```python
from build123d import *

# Parameters (mm, degrees)
BASE_FLANGE1_START             = -3.175
BASE_FLANGE1_OUTLINE_W         = 1184.91
BASE_FLANGE1_OUTLINE_H         = 203.2
BASE_FLANGE1_DEPTH             = 6.35
EDGE_FLANGE1_STRIP_W           = 48.1
EDGE_FLANGE1_STRIP_H           = 6.35
EDGE_FLANGE1_STRIP_CUT_DEPTH   = 203.2
EDGE_FLANGE1_STRIP_2_W         = 48.1
EDGE_FLANGE1_STRIP_2_H         = 6.35
EDGE_FLANGE1_STRIP_CUT_2_DEPTH = 203.2
EDGE_FLANGE1_DEPTH             = 203.2
EDGE_FLANGE1_BEND_DEPTH        = 203.2
BOSS_EXTRUDE1_START            = -6.35
BOSS_EXTRUDE1_DEPTH            = 6.35
CUT_EXTRUDE1_REACH             = 1310.867
SKETCH13_R                     = 38.1
SKETCH13_W                     = 25.908
SKETCH13_H                     = 27.94
BOSS_EXTRUDE2_DEPTH            = 6.35
MIRROR3_START                  = -165.354
MIRROR3_OUTLINE_W              = 6.35
MIRROR3_OUTLINE_H              = 27.94
MIRROR3_DEPTH                  = 25.908
MIRROR3_START_2                = 139.446
MIRROR3_2_OUTLINE_W            = 6.35
MIRROR3_2_OUTLINE_H            = 27.94
MIRROR3_2_DEPTH                = 25.908


# Read off the part's stored shape, not the designer's step: Base-Flange1, Mirror3
# Sheet-metal steps are written as plain solids
with BuildPart() as part:
    # Base-Flange1 outline → Base-Flange1 (new body)
    with BuildSketch(Plane(origin=(0, 0, 0), x_dir=(1, 0, 0), z_dir=(0, 1, 0)).offset(BASE_FLANGE1_START)):
        Rectangle(BASE_FLANGE1_OUTLINE_W, BASE_FLANGE1_OUTLINE_H)
    extrude(amount=BASE_FLANGE1_DEPTH)

    # Edge-Flange1 strip (across the edge) → Edge-Flange1 strip cut (cut)
    with BuildSketch(Plane(origin=(592.455, -3.175, -101.6), x_dir=(-1, 0, 0), z_dir=(0, 0, 1))):
        with Locations((-11.35, -3.175)):
            Rectangle(EDGE_FLANGE1_STRIP_W, EDGE_FLANGE1_STRIP_H)
    extrude(amount=EDGE_FLANGE1_STRIP_CUT_DEPTH, mode=Mode.SUBTRACT)

    # Edge-Flange1 strip 2 (across the edge) → Edge-Flange1 strip cut 2 (cut)
    with BuildSketch(Plane(origin=(-592.455, -3.175, 101.6), x_dir=(1, 0, 0), z_dir=(0, 0, -1))):
        with Locations((-11.35, -3.175)):
            Rectangle(EDGE_FLANGE1_STRIP_2_W, EDGE_FLANGE1_STRIP_2_H)
    extrude(amount=EDGE_FLANGE1_STRIP_CUT_2_DEPTH, mode=Mode.SUBTRACT)

    # Edge-Flange1 section (across the edge) → Edge-Flange1 (add)
    with BuildSketch(Plane(origin=(592.455, -3.175, -101.6), x_dir=(-1, 0, 0), z_dir=(0, 0, 1))):
        with BuildLine():
            Line((0, 6.35), (0, 514.35))
            Line((0, 514.35), (6.35, 514.35))
            Line((6.35, 514.35), (6.35, 6.35))
            ThreePointArc((6.35, 6.35), (8.209871939, 1.859871939), (12.7, 0))
            Line((12.7, 0), (12.7, -6.35))
            ThreePointArc((12.7, -6.35), (3.719743879, -2.630256121), (0, 6.35))
        make_face()
    extrude(amount=EDGE_FLANGE1_DEPTH)

    # Edge-Flange1 section 2 (across the edge) → Edge-Flange1 bend (add)
    with BuildSketch(Plane(origin=(-592.455, -3.175, 101.6), x_dir=(1, 0, 0), z_dir=(0, 0, -1))):
        with BuildLine():
            Line((0, 6.35), (0, 514.35))
            Line((0, 514.35), (6.35, 514.35))
            Line((6.35, 514.35), (6.35, 6.35))
            ThreePointArc((6.35, 6.35), (8.209871939, 1.859871939), (12.7, 0))
            Line((12.7, 0), (12.7, -6.35))
            ThreePointArc((12.7, -6.35), (3.719743879, -2.630256121), (0, 6.35))
        make_face()
    extrude(amount=EDGE_FLANGE1_BEND_DEPTH)

    # Sketch12 → Boss-Extrude1 (add)
    with BuildSketch(Plane(origin=(592.455, 0, 0), x_dir=(0, 0, -1), z_dir=(1, 0, 0)).offset(BOSS_EXTRUDE1_START)):
        Polygon((-101.6, -238.125), (-203.2, -339.725), (-203.2, -517.525), (-101.6, -517.525), align=None)
        Polygon((203.2, -339.725), (101.6, -238.125), (101.6, -517.525), (203.2, -517.525), align=None)
    extrude(amount=BOSS_EXTRUDE1_DEPTH)

    # Sketch13 → Cut-Extrude1 (cut, up to next)
    with BuildSketch(Plane(origin=(592.455, 0, 0), x_dir=(0, 0, -1), z_dir=(1, 0, 0)), mode=Mode.PRIVATE) as cut_extrude1_sk1:
        with Locations(Location((0, -73.025, 0), (0, 0, 90))):
            Circle(SKETCH13_R)
    cut_extrude1_tool1 = extrude(cut_extrude1_sk1.sketch, amount=-CUT_EXTRUDE1_REACH, mode=Mode.PRIVATE) & part.part
    # Sketch13 → Cut-Extrude1 (cut, up to next)
    with BuildSketch(Plane(origin=(592.455, 0, 0), x_dir=(0, 0, -1), z_dir=(1, 0, 0)), mode=Mode.PRIVATE) as cut_extrude1_sk2:
        with Locations((152.4, -475.107)):
            Rectangle(SKETCH13_W, SKETCH13_H)
    cut_extrude1_tool2 = extrude(cut_extrude1_sk2.sketch, amount=-CUT_EXTRUDE1_REACH, mode=Mode.PRIVATE) & part.part
    # Sketch13 → Cut-Extrude1 (cut, up to next)
    with BuildSketch(Plane(origin=(592.455, 0, 0), x_dir=(0, 0, -1), z_dir=(1, 0, 0)), mode=Mode.PRIVATE) as cut_extrude1_sk3:
        with Locations((-152.4, -475.107)):
            Rectangle(SKETCH13_W, SKETCH13_H)
    cut_extrude1_tool3 = extrude(cut_extrude1_sk3.sketch, amount=-CUT_EXTRUDE1_REACH, mode=Mode.PRIVATE) & part.part
    cut_extrude1_1 = cut_extrude1_tool1.solids().sort_by_distance((592.455, -73.025, 0))[0]
    add(cut_extrude1_1, mode=Mode.SUBTRACT)
    cut_extrude1_2 = cut_extrude1_tool2.solids().sort_by_distance((592.455, -475.107, -152.4))[0]
    add(cut_extrude1_2, mode=Mode.SUBTRACT)
    cut_extrude1_3 = cut_extrude1_tool3.solids().sort_by_distance((592.455, -475.107, 152.4))[0]
    add(cut_extrude1_3, mode=Mode.SUBTRACT)
    cut_extrude1 = cut_extrude1_1 + cut_extrude1_2 + cut_extrude1_3  # Cut-Extrude1 as one shape, for the pattern or mirror that repeats it

    # Mirror1: Cut-Extrude1 across plane
    add(cut_extrude1.mirror(Plane(origin=(0, 0, 0), x_dir=(0, 0, 1), z_dir=(1, 0, 0))), mode=Mode.SUBTRACT)

    # Sketch14 → Boss-Extrude2 (add)
    with BuildSketch(Plane.ZY.offset(592.455)):
        Polygon((203.2, -517.525), (203.2, -339.725), (101.6, -238.125), (-101.6, -238.125), (-203.2, -339.725), (-203.2, -517.525), align=None)
    extrude(amount=-BOSS_EXTRUDE2_DEPTH)

    # Mirror3 outline → Mirror3 (cut)
    with BuildSketch(Plane.XY.offset(MIRROR3_START)):
        with Locations((-589.28, -475.107)):
            Rectangle(MIRROR3_OUTLINE_W, MIRROR3_OUTLINE_H)
    extrude(amount=MIRROR3_DEPTH, mode=Mode.SUBTRACT)

    # Mirror3 2 outline → Mirror3 2 (cut)
    with BuildSketch(Plane.XY.offset(MIRROR3_START_2)):
        with Locations((-589.28, -475.107)):
            Rectangle(MIRROR3_2_OUTLINE_W, MIRROR3_2_OUTLINE_H)
    extrude(amount=MIRROR3_2_DEPTH, mode=Mode.SUBTRACT)


solid = part.part
```
Here's how the part is built. I have some questions about the finished solid (model axes, mm). A direction names the side the tool comes from. Round coordinates to 2 decimals unless told otherwise and drop trailing zeros. Order: outer loops, then holes, each group sorted by start corner. A loop starts at its lowest first (then second) coordinate and runs counter-clockwise, first axis right, second up. Notation, with made-up numbers: (-12.75, 80.5) -> (9.25, 80.5) arc R14 ccw to (9.25, 97.5) -> close; hole circle Ø9 at (43, 71.5). An arc over 180 degrees is marked (long way). Use a Markdown table: item, result. Add a question column.
(1) For pin 1 Ø3 at (x, z) = (588.5, 146) entering from +Y (3 decimals); pin 2 Ø3 at (x, z) = (207, -97) entering from -Y (3 decimals); pin 3 Ø1.9 at (x, z) = (588.5, -151) entering from +Y (3 decimals), each with a flat end and sliding along its axis, tell me the tip position at first contact or that it passes through.
(2) Suppose I cut it at D-D, the plane z = 59. Please give me the cut outline in (x, y) (3 decimals).
(3) Suppose I cut it at A-A, the plane y = -475. Please give me the cut outline in (x, z) (3 decimals), and give its area (3 significant figures).
(4) If we mould it in two halves opening along Z, with no side actions, what happens to faces 3 (the face through (589.324, -111.088, 1.675)), 4 (the face through (-8, -3.175, -1)), 5 (the face through (-589.324, -288.214, -151.689))? For each: released by +Z, released by -Z, zero draft, split by the parting line, or undercut.
(5) For faces 1 (the face through (592.455, -316, 3)), 2 (the face through (-586.105, -316, -3)), which set-ups out of +Z, -Z, +X, -X, +Y, -Y let a thin tool reach every point of the face, with its end or its side?
(6) I need wall thicknesses on line 1 along X through (y, z) = (-194.5, 17.5) (3 decimals); line 2 along Y through (x, z) = (-129.5, -78.5) (3 decimals). Which ranges of each line are inside material? Lowest first, please.
(7) Suppose I cut it at B-B, the plane z = 0. Please give me the cut outline in (x, y) (3 decimals), and give its area (3 significant figures).
(8) Suppose I cut it at C-C, the plane y = -357.5. Please give me the cut outline in (x, z) (3 decimals).
Verdict:
| question | item | result |
|---|---|---|
| 1 | pin 1 | y = -281.025 |
| 1 | pin 2 | y = -3.175 |
| 1 | pin 3 | y = -286.575 |
| 2 | outline | (-592.455, -517.525) -> (-586.105, -517.525) -> (-586.105, -9.525) arc R6.35 cw to (-579.755, -3.175) -> (579.755, -3.175) arc R6.35 cw to (586.105, -9.525) -> (586.105, -517.525) -> (592.455, -517.525) -> (592.455, -9.525) arc R12.7 ccw to (579.755, 3.175) -> (-579.755, 3.175) arc R12.7 ccw to (-592.455, -9.525) -> close |
| 3 | outline | (-592.455, -203.2) -> (-586.105, -203.2) -> (-586.105, -165.354) -> (-592.455, -165.354) -> close; (-592.455, -139.446) -> (-586.105, -139.446) -> (-586.105, 139.446) -> (-592.455, 139.446) -> close; (-592.455, 165.354) -> (-586.105, 165.354) -> (-586.105, 203.2) -> (-592.455, 203.2) -> close; (586.105, -203.2) -> (592.455, -203.2) -> (592.455, -165.354) -> (586.105, -165.354) -> close; (586.105, -139.446) -> (592.455, -139.446) -> (592.455, 139.446) -> (586.105, 139.446) -> close; (586.105, 165.354) -> (592.455, 165.354) -> (592.455, 203.2) -> (586.105, 203.2) -> close |
| 3 | area | 4,500 mm2 |
| 4 | face 3 | undercut |
| 4 | face 4 | zero draft |
| 4 | face 5 | released by -Z |
| 5 | face 1 | +Z, -Z, +X, +Y, -Y |
| 5 | face 2 | +Z, -Z, -Y |
| 6 | line 1 | -592.455 to -586.105, 586.105 to 592.455 |
| 6 | line 2 | -3.175 to 3.175 |
| 7 | outline | (-592.455, -517.525) -> (-586.105, -517.525) -> (-586.105, -111.125) -> (-592.455, -111.125) -> close; (-592.455, -34.925) -> (-586.105, -34.925) -> (-586.105, -9.525) arc R6.35 cw to (-579.755, -3.175) -> (579.755, -3.175) arc R6.35 cw to (586.105, -9.525) -> (586.105, -34.925) -> (592.455, -34.925) -> (592.455, -9.525) arc R12.7 ccw to (579.755, 3.175) -> (-579.755, 3.175) arc R12.7 ccw to (-592.455, -9.525) -> close; (586.105, -517.525) -> (592.455, -517.525) -> (592.455, -111.125) -> (586.105, -111.125) -> close |
| 7 | area | 13,000 mm2 |
| 8 | outline | (-592.455, -203.2) -> (-586.105, -203.2) -> (-586.105, 203.2) -> (-592.455, 203.2) -> close; (586.105, -203.2) -> (592.455, -203.2) -> (592.455, 203.2) -> (586.105, 203.2) -> close |
